```python
from build123d import *

# Parameters (mm, degrees)
SKETCH1_R           = 2.55
SKETCH1_R_2         = 4
SKETCH1_R_3         = 1.65
SKETCH1_R_4         = 1.75
SKETCH1_W           = 12
SKETCH1_H           = 20
SKETCH1_W_2         = 18
SKETCH1_H_2         = 3.2
SKETCH1_W_3         = 3.2
SKETCH1_H_3         = 82.4
BOSS_EXTRUDE1_DEPTH = 3


with BuildPart() as part:
    # Sketch1 → Boss-Extrude1 (new body)
    with BuildSketch(Plane(origin=(0, 0, 0), x_dir=(1, 0, 0), z_dir=(0, 1, 0))):
        Polygon((38.8, 0), (0, 0), (0, -22.5), (3, -22.5), (3, -52.5), (0, -52.5), (0, -82.5), (3, -82.5), (3, -112.5), (0, -112.5), (0, -135), (38.8, -135), (38.8, -132), (74.6, -132), (74.6, -135), (110.4, -135), (110.4, -132), (146.2, -132), (146.2, -135), (185, -135), (185, -112.5), (182, -112.5), (182, -82.5), (185, -82.5), (185, -52.5), (182, -52.5), (182, -22.5), (185, -22.5), (185, 0), (146.2, 0), (146.2, -3), (110.4, -3), (110.4, 0), (74.6, 0), (74.6, -3), (38.8, -3), align=None)
        with Locations((7.5, -128.5)):
            Circle(SKETCH1_R, mode=Mode.SUBTRACT)
        with Locations((7.5, -120.5)):
            Circle(SKETCH1_R_2, mode=Mode.SUBTRACT)
        with Locations((17, -118)):
            Circle(SKETCH1_R_3, mode=Mode.SUBTRACT)
        with Locations((54.5, -118)):
            Circle(SKETCH1_R_3, mode=Mode.SUBTRACT)
        with Locations((54.795, -105.03)):
            Circle(SKETCH1_R_4, mode=Mode.SUBTRACT)
        with Locations((17, -83.6)):
            Circle(SKETCH1_R_3, mode=Mode.SUBTRACT)
        with Locations((35.75, -67.5)):
            Rectangle(SKETCH1_W, SKETCH1_H, mode=Mode.SUBTRACT)
        with Locations((54.5, -83.6)):
            Circle(SKETCH1_R_3, mode=Mode.SUBTRACT)
        with Locations((97, -118)):
            Circle(SKETCH1_R_3, mode=Mode.SUBTRACT)
        with Locations((96.705, -105.03)):
            Circle(SKETCH1_R_4, mode=Mode.SUBTRACT)
        with Locations((134.501274191, -118)):
            Circle(SKETCH1_R_3, mode=Mode.SUBTRACT)
        with Locations((144.001274191, -128.5)):
            Circle(SKETCH1_R, mode=Mode.SUBTRACT)
        with Locations((144.001274191, -120.5)):
            Circle(SKETCH1_R_2, mode=Mode.SUBTRACT)
        with Locations((171.15, -110.3)):
            Rectangle(SKETCH1_W_2, SKETCH1_H_2, mode=Mode.SUBTRACT)
        with Locations((97, -83.6)):
            Circle(SKETCH1_R_3, mode=Mode.SUBTRACT)
        with Locations((134.5, -83.6)):
            Circle(SKETCH1_R_3, mode=Mode.SUBTRACT)
        with Locations((115.75, -67.5)):
            Rectangle(SKETCH1_W, SKETCH1_H, mode=Mode.SUBTRACT)
        with Locations((17, -51.4)):
            Circle(SKETCH1_R_3, mode=Mode.SUBTRACT)
        with Locations((54.5, -51.4)):
            Circle(SKETCH1_R_3, mode=Mode.SUBTRACT)
        with Locations((51.555, -38.93)):
            Circle(SKETCH1_R_4, mode=Mode.SUBTRACT)
        with Locations((17, -17)):
            Circle(SKETCH1_R_3, mode=Mode.SUBTRACT)
        with Locations((7.5, -14.5)):
            Circle(SKETCH1_R_2, mode=Mode.SUBTRACT)
        with Locations((7.5, -6.5)):
            Circle(SKETCH1_R, mode=Mode.SUBTRACT)
        with Locations((54.5, -17)):
            Circle(SKETCH1_R_3, mode=Mode.SUBTRACT)
        with Locations((97, -51.4)):
            Circle(SKETCH1_R_3, mode=Mode.SUBTRACT)
        with Locations((134.5, -51.4)):
            Circle(SKETCH1_R_3, mode=Mode.SUBTRACT)
        with Locations((99.945, -38.93)):
            Circle(SKETCH1_R_4, mode=Mode.SUBTRACT)
        with Locations((158.9, -67.5)):
            Rectangle(SKETCH1_W_3, SKETCH1_H_3, mode=Mode.SUBTRACT)
        with Locations((97, -17)):
            Circle(SKETCH1_R_3, mode=Mode.SUBTRACT)
        with Locations((134.5, -17)):
            Circle(SKETCH1_R_3, mode=Mode.SUBTRACT)
        with Locations((171.15, -24.7)):
            Rectangle(SKETCH1_W_2, SKETCH1_H_2, mode=Mode.SUBTRACT)
        with Locations((144, -14.5)):
            Circle(SKETCH1_R_2, mode=Mode.SUBTRACT)
        with Locations((144, -6.5)):
            Circle(SKETCH1_R, mode=Mode.SUBTRACT)
    extrude(amount=BOSS_EXTRUDE1_DEPTH)


solid = part.part
```
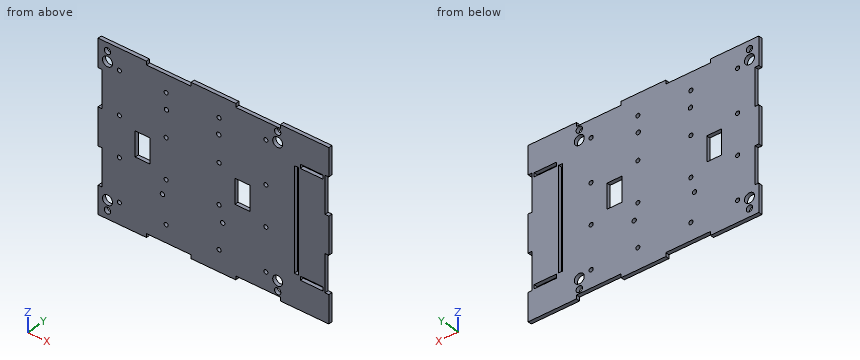
Design review of the part built by this model. Coordinates are the model's own, in mm. Give positions to 0.01 mm unless a question says otherwise; leave off trailing zeros. Loops run counter-clockwise (first coordinate to the right, second up) from the corner with the lowest first, then second, coordinate; pieces in that order, holes last. Notation, with made-up numbers: M -16.75,38 L 11.25,38 A23 cw 11.25,69 Z; hole C 75.5,23 d8. An arc over 180 degrees is marked long. Return JSON: item names as keys, results as strings. Group by question number.
Item 1: For probe 1 along Z at (x, y) = (144, 1.6); probe 2 along Z at (x, y) = (166.5, 2.3); probe 3 along Z at (x, y) = (97, 1.25), list the stretches that pass through material, from the lowest coordinate up.
Item 2: Insertion check: pin 1 Ø2.5 at (x, z) = (54.5, 83.6) entering from -Y; pin 2 Ø1.5 at (y, z) = (1.5, 111) entering from -X. Each pin has a flat end and moves straight along its axis. Give the tip position at first contact, or say it passes through.
Item 3: We need section B-B (z = 6.5). Give the boundary of the cut face in (x, y).
Item 4: We need section A-A (x = 34.5). Give the boundary of the cut face in (y, z).
Item 5: We need section C-C (x = 7.5). Give the boundary of the cut face in (y, z).
Item 6: We need section D-D (y = 1.95). Give the number of separate pieces and of enclosed holes in the cut face, and give its area (3 significant figures).
Output:
{
 "1": {"probe 1": "z = 3 to 3.95, 9.05 to 10.5, 18.5 to 116.5, 124.5 to 125.95, 131.05 to 132", "probe 2": "z = 0 to 23.1, 26.3 to 108.7, 111.9 to 135", "probe 3": "z = 0 to 15.35, 18.65 to 49.75, 53.05 to 81.95, 85.25 to 103.31, 106.75 to 116.35, 119.65 to 135"},
 "2": {"pin 1": "passes through", "pin 2": "stops at x = 3"},
 "3": {"outline": "M 0,0 L 4.95,0 L 4.95,3 L 0,3 Z; M 10.05,0 L 141.45,0 L 141.45,3 L 10.05,3 Z; M 146.55,0 L 185,0 L 185,3 L 146.55,3 Z"},
 "4": {"outline": "M 0,0 L 3,0 L 3,57.5 L 0,57.5 Z; M 0,77.5 L 3,77.5 L 3,135 L 0,135 Z"},
 "5": {"outline": "M 0,0 L 3,0 L 3,3.95 L 0,3.95 Z; M 0,9.05 L 3,9.05 L 3,10.5 L 0,10.5 Z; M 0,18.5 L 3,18.5 L 3,116.5 L 0,116.5 Z; M 0,124.5 L 3,124.5 L 3,125.95 L 0,125.95 Z; M 0,131.05 L 3,131.05 L 3,135 L 0,135 Z"},
 "6": {"separate pieces": "1", "enclosed holes": "33", "area": "22,900 mm^2"}
}
